Read the model definition and answer for the solid it produces. Units are mm, in the model's axes. Face numbers are marked on the shaded views. A direction names the side the tool comes from. Coordinates: 2 decimals unless noted, no trailing zeros. Write each loop counter-clockwise with the first axis right and the second up, starting at its lowest first coordinate (ties: lowest second). Pieces come first, ordered by that corner, then holes.
(1) The part is cut by section A-A, the plane y = 8. Determine the outline of the cut face in (x, z) (3 decimals).
(2) The part is cut by section C-C, the plane y = -12. Determine the outline of the cut face in (x, z) (3 decimals).
(3) Determine the mould class of the marked faces 3, 4 and 5 for opening direction X: pulls with the +X half, pulls with the -X half, needs draft (parallel to the pull), parting line crosses it, or undercut.
(4) The part is cut by section B-B, the plane z = 9. Determine the outline of the cut face in (x, y) (3 decimals), and give its area (3 significant figures).
(5) Given pin 1 (4 mm diameter, centred on x = -6, z = -6.5, fed in from -Y), flat-ended and moving along its own axis, determine where the tip first touches the part or whether it passes through.
(6) Straight lines are drawn through the part: line 1 along Z through (x, y) = (10.55, 0); line 2 along Z through (x, y) = (9.75, -5.5); line 3 along X through (y, z) = (-5, -11.5) (3 decimals). For each, find the intervals that lie inside material, in ascending order.
(7) Which of the six approach directions +Z, -Z, +X, -X, +Y, -Y give full straight-line access (tool end or side, diameter ignored) to the marked faces 1 and 2?
(8) The part is cut by section D-D, the plane x = 10.5. State how many separate pieces and enclosed holes the cut face has, and give its area (3 significant figures).
```python
from build123d import *

# Parameters (mm, degrees)
F0_W     = 2.54
F0_H     = 10.16
F0_H_2   = 5.08
F0_W_2   = 19.05
F2_R     = 4
F2_R_2   = 1.85
F3_DEPTH = 25.4


with BuildPart() as f1:
    # F0 (on Top) → F1 (revolve)
    with BuildSketch(Plane.XY):
        with Locations((-10.795, 10.16)):
            Rectangle(F0_W, F0_H)
        with Locations((-10.795, 2.54)):
            Rectangle(F0_W, F0_H_2)
        with Locations((0, 2.54)):
            Rectangle(F0_W_2, F0_H_2)
        Polygon((9.525, 15.24), (9.525, 5.08), (9.525, 0), (12.065, 0), (12.065, 15.24), align=None)
    revolve(axis=Axis((0, 0, 0), (1, 0, 0)))

    # F2 (on face) → F3 (cut)
    with BuildSketch(Plane.YZ.offset(12.065)):
        Circle(F2_R)
        with Locations((0, 8)):
            Circle(F2_R_2)
        with Locations((-5.656854, 5.656854)):
            Circle(F2_R_2)
        with Locations((-8, 0)):
            Circle(F2_R_2)
        with Locations((-5.656854, -5.656854)):
            Circle(F2_R_2)
        with Locations((0, -8)):
            Circle(F2_R_2)
        with Locations((5.656854, -5.656854)):
            Circle(F2_R_2)
        with Locations((8, 0)):
            Circle(F2_R_2)
        with Locations((5.656854, 5.656854)):
            Circle(F2_R_2)
    extrude(amount=-F3_DEPTH, mode=Mode.SUBTRACT)


solid = f1.part
```
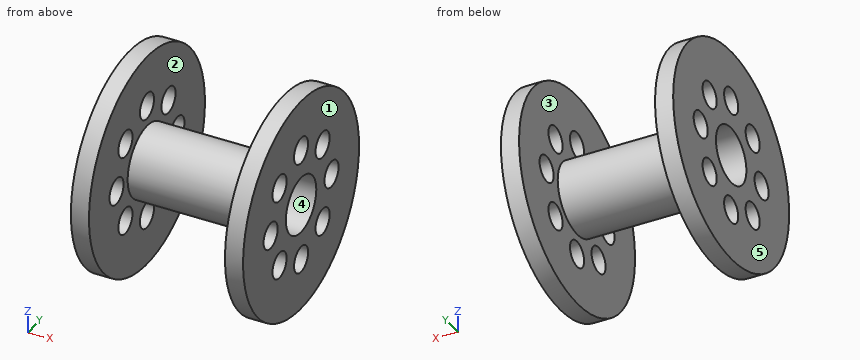
Computed:
1. outline: (-12.065, -12.971) - (-9.525, -12.971) - (-9.525, -1.85) - (-12.065, -1.85) - close; (-12.065, 1.85) - (-9.525, 1.85) - (-9.525, 12.971) - (-12.065, 12.971) - close; (9.525, -12.971) - (12.065, -12.971) - (12.065, -1.85) - (9.525, -1.85) - close; (9.525, 1.85) - (12.065, 1.85) - (12.065, 12.971) - (9.525, 12.971) - close
2. outline: (-12.065, -9.395) - (-9.525, -9.395) - (-9.525, 9.395) - (-12.065, 9.395) - close; (9.525, -9.395) - (12.065, -9.395) - (12.065, 9.395) - (9.525, 9.395) - close
3. face 3: undercut
3. face 4: needs draft
3. face 5: pulls with the -X half
4. outline: (-12.065, -12.299) - (-9.525, -12.299) - (-9.525, -1.556) - (-12.065, -1.556) - close; (-12.065, 1.556) - (-9.525, 1.556) - (-9.525, 12.299) - (-12.065, 12.299) - close; (9.525, -12.299) - (12.065, -12.299) - (12.065, -1.556) - (9.525, -1.556) - close; (9.525, 1.556) - (12.065, 1.556) - (12.065, 12.299) - (9.525, 12.299) - close
4. area: 109 mm2
5. pin 1: stops at y = -2.36
6. line 1: z = -15.24 to -9.85, -6.15 to -4, 4 to 6.15, 9.85 to 15.24
6. line 2: z = -14.21 to -7.5, -3.81 to 3.81, 7.5 to 14.21
6. line 3: x = -12.065 to -9.525, 9.525 to 12.065
7. face 1: +Z, -Z, +X, +Y, -Y
7. face 2: none
8. separate pieces: 1
8. enclosed holes: 9
8. area: 593 mm2
